Work out the finished part from the listing and answer in its coordinate system (mm). Coordinates: 2 decimals unless noted, no trailing zeros. Order: outer loops, then holes, each group sorted by start corner. A loop starts at its lowest first (then second) coordinate and runs counter-clockwise, first axis right, second up. Notation, with made-up numbers: M 48.5,61.5 L 53.5,61.5 A17 ccw 53.5,83.5 Z; hole C -29.75,-29 d8. An arc over 180 degrees is marked long. Use a Markdown table: item, result.
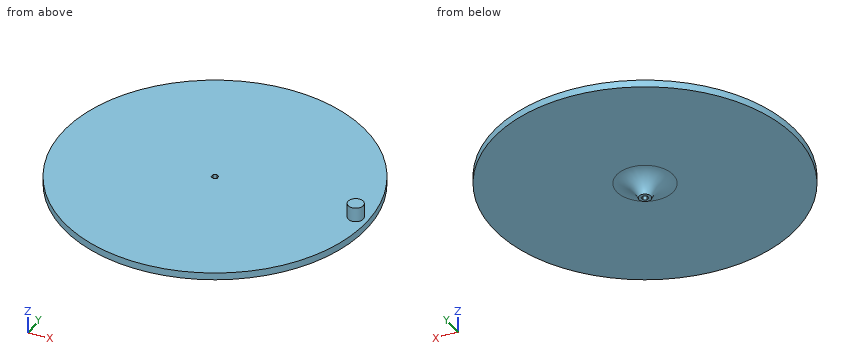
from build123d import *

# Parameters (mm, degrees)
SKETCH1_R           = 63.5
BOSS_EXTRUDE1_DEPTH = 3
SKETCH3_R           = 3.175
BOSS_EXTRUDE2_DEPTH = 6
CUT_EXTRUDE1_DEPTH  = 6
SKETCH5_R           = 2.5
BOSS_EXTRUDE3_DEPTH = 6.5
FILLET1_R           = 10


with BuildPart() as part:
    # Sketch1 → Boss-Extrude1 (new body)
    with BuildSketch(Plane.XY):
        Circle(SKETCH1_R)
    extrude(amount=BOSS_EXTRUDE1_DEPTH)

    # Sketch3 → Boss-Extrude2 (add)
    with BuildSketch(Plane.XY.offset(3)):
        with Locations((58.325, 0)):
            Circle(SKETCH3_R)
    extrude(amount=BOSS_EXTRUDE2_DEPTH)

    # Sketch4 → Cut-Extrude1 (cut)
    with BuildSketch(Plane.XY.offset(3)):
        Polygon((0, 1.443375673), (-1.25, 0.721687836), (-1.25, -0.721687836), (0, -1.443375673), (1.25, -0.721687836), (1.25, 0.721687836), align=None)
    extrude(amount=-CUT_EXTRUDE1_DEPTH, mode=Mode.SUBTRACT)

    # Sketch5 → Boss-Extrude3 (add)
    with BuildSketch(Plane(origin=(0, 0, 0), x_dir=(-1, 0, 0), z_dir=(0, 0, -1))):
        with Locations(Location((0, 0, 0), (0, 0, 180))):
            Circle(SKETCH5_R)
        Polygon((-1.25, 0.721687836), (0, 1.443375673), (1.25, 0.721687836), (1.25, -0.721687836), (0, -1.443375673), (-1.25, -0.721687836), align=None, mode=Mode.SUBTRACT)
    extrude(amount=BOSS_EXTRUDE3_DEPTH)

    # Fillet1
    # the kernel refuses this fillet: 10 mm, written as the material it adds along each edge
    with BuildSketch(Plane(origin=(0, 0, 0), x_dir=(1, 0, 0), z_dir=(0, 1, 0))) as fillet1_piece_1:
        with BuildLine():
            CenterArc((11.867496998, 10), FILLET1_R, 200.487315115, 69.512684885)
            Line((11.867496998, 0), (11.867496998, -0.2))
            Line((11.867496998, -0.2), (2.5, -0.2))
            Line((2.5, -0.2), (2.3, 0))
            ThreePointArc((2.3, 0), (2.3, 3.25), (2.31265006, 6.43))
            Line((2.31265006, 6.43), (2.5, 6.5))
        make_face()
    revolve(axis=Axis((0, 0, 0), (0, 0, -1)))


solid = part.part
1. Section A-A on z = -3 is taken. Determine the outline of the cut face in (x, y), then the cut area to 3 significant figures.
Answers below:
| item | result |
|---|---|
| outline | C 0,0 d9.45; hole M -1.25,-0.72 L 0,-1.44 L 1.25,-0.72 L 1.25,0.72 L 0,1.44 L -1.25,0.72 Z |
| area | 64.8 mm² |
2. Find the intervals of material crossed by probe 1 along Z at (x, y) = (28.5, -20); probe 2 along Y at (x, z) = (-44, 1); probe 3 along Y at (x, z) = (3, -1.5), in increasing order.
Answers below:
| item | result |
|---|---|
| probe 1 | 0 to 3 |
| probe 2 | -45.78 to 45.78 |
| probe 3 | -5.88 to 5.88 |
3. Section B-B on z = 7 is taken. Determine the outline of the cut face in (x, y) (3 decimals), then the cut area to 3 significant figures.
Answers below:
| item | result |
|---|---|
| outline | C 58.325,0 d6.35 |
| area | 31.7 mm² |
4. Section D-D on x = 19 is taken. Determine the outline of the cut face in (y, z), then the cut area to 3 significant figures.
Answers below:
| item | result |
|---|---|
| outline | M -60.59,0 L 60.59,0 L 60.59,3 L -60.59,3 Z |
| area | 364 mm² |
5. Section C-C on y = 30 is taken. Determine the outline of the cut face in (x, z).
Answers below:
| item | result |
|---|---|
| outline | M -55.97,0 L 55.97,0 L 55.97,3 L -55.97,3 Z |
6. Flat-ended cylindrical pins translate along their axes: P1, Ø4, axis at y = -15, z = 2, coming from the +X side; P2, Ø4, axis at x = -32, y = 27.5, coming from the +Z side; P3, Ø8, axis at y = 39, z = -3.5, coming from the +X side; P4, Ø3, axis at x = 13, z = 6, coming from the -Y side (1 decimal). Find the tip coordinate at first contact, or state that the pin passes through.
Answers below:
| item | result |
|---|---|
| P1 | x = 62.16 |
| P2 | z = 3 |
| P3 | x = 51.56 |
| P4 | through |
